Part model, mm, in its own coordinate system. A direction names the side the tool comes from. Coordinates: 2 decimals unless noted, no trailing zeros. Write each loop counter-clockwise with the first axis right and the second up, starting at its lowest first coordinate (ties: lowest second). Pieces come first, ordered by that corner, then holes. Notation, with made-up numbers: (77.25, 45) - (119.25, 45) arc R23 ccw to (119.25, 62) - close; hole circle Ø10 at (-27.75, 42). An arc over 180 degrees is marked (long way). Use a Markdown table: item, result.
```python
from build123d import *

# Parameters (mm, degrees)
CHAMFER1_SIZE      = 0.29
CHAMFER1_SIZE2     = 0.502294734
CUT_EXTRUDE1_DEPTH = 1.5
DRAFT1_ANGLE       = 35
DRAFT2_ANGLE       = 8


with BuildPart() as part:
    # Sketch1 → Revolve1 (revolve)
    with BuildSketch(Plane.XY, mode=Mode.PRIVATE) as revolve1_sk:
        Polygon((0, 2.75), (0.4, 2.75), (1.7, 1.45), (6.5, 1.45), (6.5, 0), (0, 0), align=None)
    revolve(revolve1_sk.sketch.rotate(Axis((6.620684694, 0, 0), (-1, 0, 0)), 90), axis=Axis((6.620684694, 0, 0), (-1, 0, 0)))

    # Chamfer1
    chamfer1_edges = [part.edges().sort_by_distance(p)[0] for p in [
        (6.5, 0, 1.45),
    ]]
    chamfer1_side = [part.faces().sort_by_distance(p)[0] for p in [
        (6.5, 0, 0),
    ]]
    chamfer(chamfer1_edges, length=CHAMFER1_SIZE, length2=CHAMFER1_SIZE2, reference=chamfer1_side[0])

    # Sketch3 → EndCone (revolve, cut)
    with BuildSketch(Plane.XY, mode=Mode.PRIVATE) as endcone_sk:
        Polygon((4.55, 1.45), (6.5, 1.45), (6.7, 1.45), (6.7, 0), (6.5, 0), align=None)
    revolve(endcone_sk.sketch.rotate(Axis((2.9, 0, 0), (1, 0, 0)), 270), axis=Axis((2.9, 0, 0), (1, 0, 0)), mode=Mode.SUBTRACT)

    # Sketch4 → Cut-Extrude1 (cut)
    with BuildSketch(Plane.ZY):
        Polygon((-0.4, 1.6), (-0.4, 0.4), (-1.6, 0.4), (-1.6, -0.4), (-0.4, -0.4), (-0.4, -1.6), (0.4, -1.6), (0.4, -0.4), (1.6, -0.4), (1.6, 0.4), (0.4, 0.4), (0.4, 1.6), align=None)
    extrude(amount=-CUT_EXTRUDE1_DEPTH, mode=Mode.SUBTRACT)

    # Draft1
    draft1_faces = [part.faces().sort_by_distance(p)[0] for p in [
        (0.75, 0, 1.6),
        (0.75, 1.6, 0),
        (0.75, 0, -1.6),
        (0.75, -1.6, 0),
    ]]
    draft(draft1_faces, Plane(origin=(0, 0, 0), x_dir=(0, 0, -1), z_dir=(-1, 0, 0)), DRAFT1_ANGLE)

    # Draft2
    draft2_faces = [part.faces().sort_by_distance(p)[0] for p in [
        (0.555453044, -0.805533796, -0.4),
        (0.555453044, -0.4, -0.805533796),
        (0.555453044, -0.4, 0.805533796),
        (0.555453044, -0.805533796, 0.4),
        (0.555453044, 0.805533796, 0.4),
        (0.555453044, 0.4, 0.805533796),
        (0.555453044, 0.4, -0.805533796),
        (0.555453044, 0.805533796, -0.4),
    ]]
    draft(draft2_faces, Plane(origin=(0, 0, 0), x_dir=(0, 0, -1), z_dir=(-1, 0, 0)), DRAFT2_ANGLE)

    # Sketch6 for Cut-Loft1 → Cut-Loft1 section 0
    with BuildSketch(Plane.ZY.offset(-1.5)):
        with BuildLine():
            Line((-0.36943872, 0.189188748), (-0.36943872, -0.189188748))
            # circular arc as an exact rational Bezier (weights 1, cos(half-angle), 1)
            Bezier((-0.36943872, -0.189188748), (-0.189188748, -0.189188748), (-0.189188748, -0.36943872), weights=[1, 0.707106781, 1])
            Line((-0.189188748, -0.36943872), (0.189188748, -0.36943872))
            Bezier((0.189188748, -0.36943872), (0.189188748, -0.189188748), (0.36943872, -0.189188748), weights=[1, 0.707106781, 1])
            Line((0.36943872, -0.189188748), (0.36943872, 0.189188748))
            Bezier((0.36943872, 0.189188748), (0.189188748, 0.189188748), (0.189188748, 0.36943872), weights=[1, 0.707106781, 1])
            Line((0.189188748, 0.36943872), (-0.189188748, 0.36943872))
            Bezier((-0.189188748, 0.36943872), (-0.189188748, 0.189188748), (-0.36943872, 0.189188748), weights=[1, 0.707106781, 1])
        make_face()
    # Sketch7 for Cut-Loft1 → Cut-Loft1 section 1
    with BuildSketch(Plane.ZY):
        with BuildLine():
            Line((0.580249972, 0.4), (0.580249972, -0.4))
            Bezier((0.580249972, -0.4), (0.4, -0.4), (0.4, -0.580249972), weights=[1, 0.707106781, 1])
            Line((0.4, -0.580249972), (-0.4, -0.580249972))
            Bezier((-0.4, -0.580249972), (-0.4, -0.4), (-0.580249972, -0.4), weights=[1, 0.707106781, 1])
            Line((-0.580249972, -0.4), (-0.580249972, 0.4))
            Bezier((-0.580249972, 0.4), (-0.4, 0.4), (-0.4, 0.580249972), weights=[1, 0.707106781, 1])
            Line((-0.4, 0.580249972), (0.4, 0.580249972))
            Bezier((0.4, 0.580249972), (0.4, 0.4), (0.580249972, 0.4), weights=[1, 0.707106781, 1])
        make_face()
    loft(mode=Mode.SUBTRACT)


solid = part.part
```
Item 1: Band-saw the part on B-B, the plane x = 5. Give the cut face in (y, z).
From the geometry:
| item | result |
|---|---|
| outline | circle Ø2.23 at (0, 0) |
Item 2: Band-saw the part on A-A, the plane x = 3.5. Give the cut face in (y, z).
From the geometry:
| item | result |
|---|---|
| outline | circle Ø2.9 at (0, 0) |
Item 3: Two-plate mould, pull along Z, no slides. Class faces 4 (the face through (0.57, -0.01, 1.2)), 5 (the face through (5.94, -0.25, 0.33)), 6 (the face through (0, 1, 1)): pulls with the +Z half, pulls with the -Z half, needs draft (parallel to the pull), parting line crosses it, or undercut.
From the geometry:
| item | result |
|---|---|
| face 4 | undercut |
| face 5 | parting line crosses it |
| face 6 | needs draft |
Item 4: Drill centre lines: probe 1 along Z at (x, y) = (1, -0.05); probe 2 along Y at (x, z) = (0.5, 1.2); probe 3 along X at (y, z) = (-1.15, 0.5). Where is each one in solid material? Low to high.
From the geometry:
| item | result |
|---|---|
| probe 1 | -2.15 to -0.9, 0.9 to 2.15 |
| probe 2 | -2.36 to -0.33, 0.33 to 2.36 |
| probe 3 | 0 to 4.81 |
Item 5: Which spindle directions (+Z, -Z, +X, -X, +Y, -Y) get a long thin tool onto all of the face, cutting with end or side? Do faces 1 (the face through (0.57, 0.32, 0.86)), 2 (the face through (0.203, 2.685, 0.596)), 3 (the face through (3.14, -0.06, 1.45)). Say none if no direction does.
From the geometry:
| item | result |
|---|---|
| face 1 | -X |
| face 2 | +X, -X |
| face 3 | +X |
Item 6: Drop flat-ended pins along their axis: P1, Ø3, axis at x = 4, z = 1.5, coming from the -Y side; P2, Ø1, axis at x = 1.5, y = -1, coming from the -Z side; P3, Ø1.5, axis at x = 1.5, z = 1, coming from the +Y side. Give the stop position or say it passes through.
From the geometry:
| item | result |
|---|---|
| P1 | y = -1.45 |
| P2 | z = -1.95 |
| P3 | y = 2.23 |
